Input: dimensioned drawing with shaded views. Units: mm. Origin: part minimum x, y, z. Coordinates: 2 decimals unless noted, no trailing zeros. Order: outer loops, then holes, each group sorted by start corner. A loop starts at its lowest first (then second) coordinate and runs counter-clockwise, first axis right, second up. Notation, with made-up numbers: (-32.5, 49.25) - (2.5, 49.25) arc R25 cw to (2.5, 84.25) - close; hole circle Ø11 at (-27, 8.25). An arc over 180 degrees is marked (long way). Answer as CSV lines item,"result". Start each with the question number.
Item 1: Section C-C (y = 149.5). Output: boundary loops of the cut face in (x, z), and give its area (3 significant figures).
Item 2: Material intervals for line 1 along Z through (x, y) = (17.25, 429.5); line 2 along Z through (x, y) = (17.5, 123.5), sorted ascending.
Item 3: Section A-A (x = 14.5). Output: boundary loops of the cut face in (y, z), and give its area (3 significant figures).
Item 4: Section B-B (z = 86). Output: boundary loops of the cut face in (x, y).
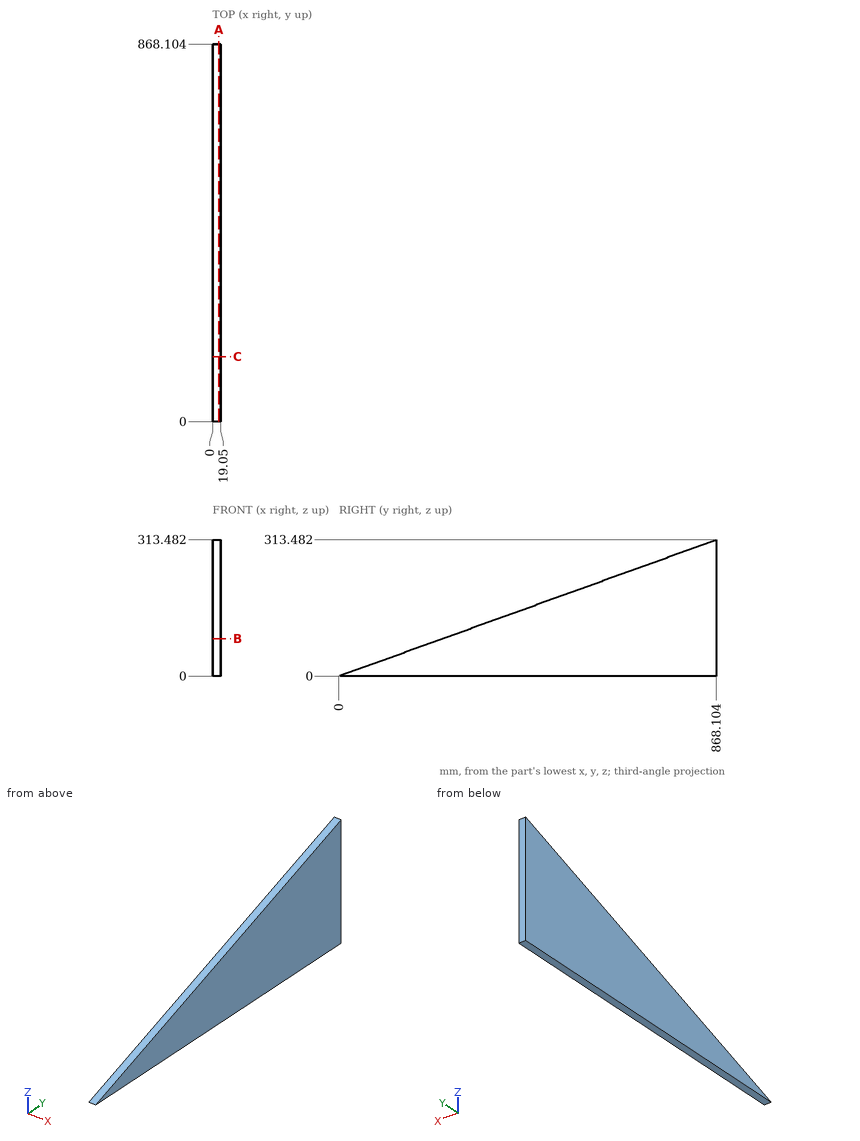
Determined:
1,outline,"(0, 0) - (19.05, 0) - (19.05, 53.99) - (0, 53.99) - close"
1,area,"1,030 mm^2"
2,line 1,"z = 0 to 155.1"
2,line 2,"z = 0 to 44.6"
3,outline,"(0, 0) - (868.1, 0) - (868.1, 313.48) - close"
3,area,"136,000 mm^2"
4,outline,"(0, 238.15) - (19.05, 238.15) - (19.05, 868.1) - (0, 868.1) - close"
